Check sheet for the modelled part. Datum: model origin and axes. Units: mm. Face numbers are marked on the shaded views. A direction names the side the tool comes from. Round coordinates to 2 decimals unless told otherwise and drop trailing zeros. Order: outer loops, then holes, each group sorted by start corner. A loop starts at its lowest first (then second) coordinate and runs counter-clockwise, first axis right, second up.
(1) Mould release check, pull along X, two halves, no side actions. Record for the marked faces 3, 4 and 5: released by +X, released by -X, zero draft, split by the parting line, or undercut.
(2) Sectioned sample at A-A, the plane y = 6.25. Enter the section's corners in (x, z), and give its area (3 significant figures).
(3) Thickness scan on probe 1 along X at (y, z) = (2.5, -17); probe 2 along Y at (x, z) = (28.25, -22.5); probe 3 along X at (y, z) = (0.75, -21.75). Record the ranges inside material, lowest first.
(4) Sectioned sample at B-B, the plane z = -7.75. Enter the section's corners in (x, y).
(5) Depth check by flat-ended pin: pin 1 (4.5 mm diameter, centred on x = 23.5, z = -9, fed in from +Y); pin 2 (1 mm diameter, centred on y = 0.5, z = -18, fed in from +X); pin 3 (0.6 mm diameter, centred on x = 31, z = -19, fed in from -Y). Enter the tip coordinate at first touch or a pass-through.
(6) Tool access check on the marked faces 1 and 2. Record the directions out of +Z, -Z, +X, -X, +Y, -Y that give a thin tool (end or side, any length) a straight path to the whole face; none if there is none.
(7) Sectioned sample at C-C, the plane x = 25.75. Enter the section's corners in (y, z).
(8) Sectioned sample at D-D, the plane z = -22. Enter the section's corners in (x, y), and give its area (3 significant figures).
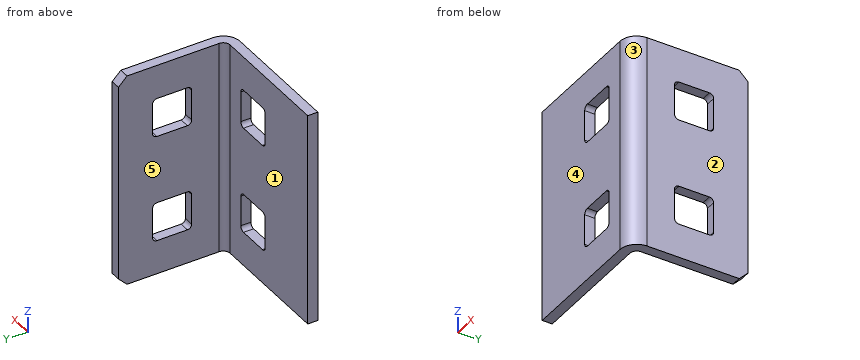
Autodesk Inventor part; units mm, degrees
ref_plane "Flange Pattern Plane" through (31.75, 7.5406, -4.5466) normal (0, 1, 0) x (1, 0, 0)
ref_plane "YZ Plane" through (0, 0, 0) normal (1, 0, 0) x (0, 1, 0)
ref_plane "XZ Plane" through (0, 0, 0) normal (0, 1, 0) x (-1, 0, 0)
sketch "Sketch1" plane through (0, 0, 0) normal (0, 1, 0) x (-1, 0, 0)
  line L0 (-31.75, 0) -> (31.75, 0)
  line L1 (31.75, 0) -> (31.75, -25.4)
  line L2 (31.75, -25.4) -> (-31.75, -25.4)
  line L3 (-31.75, -25.4) -> (-31.75, 0)
  line L4 (31.75, 0) -> (-31.75, -25.4) construction
  point P0 (0, 0)
  point P1 (0, 0)
  dimension "d0" = 63.5
  dimension "d1" = 25.4
extrude "Plate1" add sketch "Sketch1" along normal blind 1.1906
sketch "Sketch2" plane through (30.5594, 0, -25.4) normal (1, 0, 0) x (0, 1, 0)
  line L0 (0, 25.4) -> (0, 0)
  line L1 (0, 0) -> (13.8906, 0)
  line L2 (13.8906, 0) -> (13.8906, 25.4)
  line L3 (13.8906, 25.4) -> (0, 25.4)
edge flange "Flanges" height 12.7 angle 90 thickness 1.1906 bend radius 0.7937 thickness toward (1, 0, 0) relief tear relief width 1.1906 relief depth 0.5953 corner gap 1.1906 corner form 0 edges at (31.75, 1.1906, -12.7) (-31.75, 1.1906, -12.7) wall of the first edge with corners at (30.5594, 0, 0) (30.5594, 0, -25.4) (30.5594, 13.8906, -25.4) (30.5594, 13.8906, 0)
bend "Bend1"
corner "Corner1"
sketch "Sketch3" plane through (31.75, 1.9844, -25.4) normal (1, 0, 0) x (0, 0, -1)
  line L0 (-20.8534, 7.8676) -> (-17.2466, 7.8676)
  line L1 (-16.7386, 7.3596) -> (-16.7386, 3.7528)
  line L2 (-17.2466, 3.2448) -> (-20.8534, 3.2448)
  line L3 (-21.3614, 3.7528) -> (-21.3614, 7.3596)
  arc A0 (-20.8534, 7.8676) -> (-21.3614, 7.3596) centre (-20.8534, 7.3596) ccw
  arc A1 (-16.7386, 7.3596) -> (-17.2466, 7.8676) centre (-17.2466, 7.3596) ccw
  arc A2 (-17.2466, 3.2448) -> (-16.7386, 3.7528) centre (-17.2466, 3.7528) ccw
  arc A3 (-21.3614, 3.7528) -> (-20.8534, 3.2448) centre (-20.8534, 3.7528) ccw
  line L4 (-25.4, 0) -> (-25.4, 11.9062) construction
  line L5 (-25.4, 11.9062) -> (0, 11.9063) construction
  line L6 (-20.8534, 7.3596) -> (-17.2466, 3.7528) construction
  point P0 (-25.4, -1.9844)
  point P1 (-16.7386, 3.2448)
  point P2 (-21.3614, 3.2448)
  point P3 (-19.05, 5.5562)
  dimension "d16" = 4.6228
  dimension "d17" = 0.508
  dimension "d20" = 6.35
  dimension "d21" = 6.35
extrude "Flange Stamp" cut sketch "Sketch3" against normal blind 1.1906
sketch "Sketch7" plane through (31.75, 1.9844, 0) normal (1, 0, 0) x (0, 0, -1)
  arc A0 (4.5466, 7.8676) -> (4.0386, 7.3596) centre (4.5466, 7.3596) ccw construction
  arc A1 (8.1534, 3.2448) -> (8.6614, 3.7528) centre (8.1534, 3.7528) ccw construction
  circle A2 centre (6.35, 5.5563) radius 2.1844
  line L0 (4.5466, 7.3596) -> (8.1534, 3.7528) construction
  point P0 (0, -1.9844)
  dimension "d46" = 4.3688
surface extrude "Flange Circle" sketch "Sketch7" against normal up to surface (1.1906 mm away) shown yes curves A2
ref_plane "Flange Pattern Plane" through (31.75, 7.5406, -4.5466) normal (0, 1, 0) x (1, 0, 0)
sketch "Flange Pattern Sketch" plane through (31.75, 7.5406, -4.5466) normal (0, 1, 0) x (1, 0, 0)
  line L0 (0, 3.6068) -> (0, 0) construction
  line L1 (-76.2822, -4.5466) -> (13.1932, -4.5466) construction
  line L2 (0, 0) -> (-1.1906, 0) construction
  point P0 (-31.75, -4.5466)
  point P1 (0, 1.8034)
  point P2 (0, 14.5034)
  dimension "d131" = 12.7
  dimension "d134" = 12.7
pattern_sketch "Flange Pattern" of "Flange Circle", "Flange Stamp" from (31.75, 7.5406, -6.35) copies at (31.75, 7.5406, -19.05)
sketch "Sketch8" plane through (0, 0, 0) normal (0, -1, 0) x (1, 0, 0)
  line L0 (29.7656, 0) -> (-29.7656, 0) construction
  line L1 (27.2034, -4.0386) -> (23.5966, -4.0386)
  line L2 (23.0886, -4.5466) -> (23.0886, -8.1534)
  line L3 (23.5966, -8.6614) -> (27.2034, -8.6614)
  line L4 (27.7114, -8.1534) -> (27.7114, -4.5466)
  arc A0 (27.7114, -4.5466) -> (27.2034, -4.0386) centre (27.2034, -4.5466) ccw
  arc A1 (27.2034, -8.6614) -> (27.7114, -8.1534) centre (27.2034, -8.1534) ccw
  arc A2 (23.0886, -8.1534) -> (23.5966, -8.6614) centre (23.5966, -8.1534) ccw
  arc A3 (23.5966, -4.0386) -> (23.0886, -4.5466) centre (23.5966, -4.5466) ccw
  line L5 (27.2034, -4.5466) -> (23.5966, -8.1534) construction
  line L6 (31.75, 0) -> (31.75, -25.4) construction
  point P0 (0, 0)
  point P1 (23.0886, -8.6614)
  point P2 (27.7114, -8.6614)
  point P3 (25.4, -6.35)
  dimension "d49" = 4.6228
  dimension "d50" = 0.508
  dimension "d51" = 6.35
  dimension "d52" = 6.35
extrude "Body Stamp" cut sketch "Sketch8" against normal blind 1.1906
sketch "Sketch9" plane through (0, 0, 0) normal (0, -1, 0) x (1, 0, 0)
  arc A0 (27.7114, -4.5466) -> (27.2034, -4.0386) centre (27.2034, -4.5466) ccw construction
  arc A1 (23.0886, -8.1534) -> (23.5966, -8.6614) centre (23.5966, -8.1534) ccw construction
  line L0 (27.2034, -4.5466) -> (23.5966, -8.1534) construction
  circle A2 centre (25.4, -6.35) radius 2.1844
  point P0 (0, 0)
  dimension "d55" = 4.3688
surface extrude "Body Circle" sketch "Sketch9" against normal up to surface (1.1906 mm away) shown yes curves A2
sketch "Body Pattern Sketch" plane through (0, 0, 0) normal (0, -1, 0) x (1, 0, 0)
  line L0 (29.7656, 0) -> (-29.7656, 0) construction
  line L1 (31.75, 0) -> (31.75, -25.4) construction
  circle A0 centre (25.4, -6.35) radius 2.1844 construction
  point P0 (0, 0)
  point P1 (25.4, -19.05)
  dimension "d62" = 12.7
  dimension "d65" = 12.7
  dimension "d139" = 12.7
pattern_sketch "Body Pattern" of "Body Stamp", "Body Circle" from (25.4, 0, -6.35) copies at (25.4, 0, -19.05)
sketch "Arc Length" plane through (30.5594, 1.9844, 0) normal (0, 0, 1) x (1, 0, 0)
  line L0 (0, 0) -> (1.1906, 0) construction
  arc A0 (-0.7938, -0.7938) -> (0, 0) centre (-0.7938, 0) ccw construction
  line L1 (-0.7938, -1.9844) -> (-0.7938, -0.7938) construction
  arc A1 (-0.7938, -1.9844) -> (1.1906, 0) centre (-0.7938, 0) ccw construction
  point P0 (-30.5594, -1.9844)
  dimension "d85" = 3.117
  dimension "d92" = 1.2468
sketch "Sketch13" plane through (31.75, 13.8906, 0) normal (1, 0, 0) x (0, 0, -1)
  line L0 (0, 0) -> (25.4, 0) construction
  line L1 (62.4078, 0) -> (63.4238, -1.016)
  line L2 (63.4238, -1.016) -> (64.4398, 0)
  line L3 (62.4078, 0) -> (64.4398, 0)
  line L4 (25.4, -11.9063) -> (0, -11.9063) construction
  line L5 (63.4238, -10.8903) -> (61.3168, -12.9972)
  line L6 (61.3168, -12.9972) -> (63.4238, -15.1042)
  line L7 (63.4238, -15.1042) -> (65.5308, -12.9972)
  line L8 (65.5308, -12.9972) -> (63.4238, -10.8903)
  line L9 (63.4238, -10.8903) -> (63.4238, -15.1042) construction
  line L10 (63.4238, -1.016) -> (63.4238, -10.8903) construction
  line L11 (0, -11.9063) -> (25.4, -11.9063) construction
  point P0 (0, -13.8906)
  dimension "d86" = 4.2139
  dimension "d88" = 1.016
  dimension "d91" = 1.016
  dimension "d102" = 63.4238
feature "Notch" [suppressed]
mirror "Notch Mirror" [suppressed]
pattern_linear "Notch Pattern" [suppressed]
chamfer "End Chamfer" distance 1.016 angle 45 4 edges at (-31.1547, 13.8906, -25.4) (31.1547, 13.8906, -25.4) (-31.1547, 13.8906, 0) (31.1547, 13.8906, 0)
sketch "Sketch14" plane through (-31.75, 1.9844, 419.1) normal (1, 0, 0) x (0, 0, -1)
  line L0 (419.1, 11.9063) -> (444.5, 11.9063) construction
  line L1 (419.1, 0) -> (419.1, 11.9063) construction
  line L2 (419.1, -1.9844) -> (444.5, -1.9844) construction
  line L3 (419.1, 11.9063) -> (444.5, 11.9063)
  line L4 (444.5, 11.9063) -> (444.5, -1.9844)
  line L5 (444.5, -1.9844) -> (419.1, -1.9844)
  line L6 (419.1, -1.9844) -> (419.1, 11.9063)
  point P0 (382.0521, -1.9844)
extrude "Half Cut" cut sketch "Sketch14" along normal blind 46.7614
equation "\"d1\" = 1.27 * Length"
equation "\"d18\" = Thickness"
equation "\"d53\" = Thickness"
equation "\"d89\" = Thickness"
equation "\"d2\" = Thickness"
equation "\"d3\" = BendReliefWidth"
equation "\"d4\" = BendReliefDepth"
equation "\"d5\" = MinimumRemnant"
equation "\"d6\" = TransitionRadius"
equation "\"d10\" = CornerReliefSize"
equation "\"d11\" = GapSize"
equation "\"d12\" = JacobiRadiusSize"
equation "\"BendRadius\" = Thickness"
equation "\"BendReliefWidth\" = Thickness"
equation "\"BendReliefDepth\" = 0.5 * Thickness"
equation "\"CornerReliefSize\" = 4 * Thickness"
equation "\"MinimumRemnant\" = 2 * Thickness"
equation "\"TransitionRadius\" = BendRadius"
equation "\"JacobiRadiusSize\" = BendRadius"
equation "\"GapSize\" = Thickness"
properties part number "Alu C 1x3x1x35"
Derived:
1. face 3: released by +X
1. face 4: zero draft
1. face 5: released by -X
2. outline: (30.56, -25.4) - (31.75, -25.4) - (31.75, -21.36) - (30.56, -21.36) - close; (30.56, -16.74) - (31.75, -16.74) - (31.75, -8.66) - (30.56, -8.66) - close; (30.56, -4.04) - (31.75, -4.04) - (31.75, 0) - (30.56, 0) - close
2. area: 19.2 mm2
3. probe 1: x = 30.56 to 31.75
3. probe 2: y = 0 to 1.19
3. probe 3: x = 15.01 to 31.32
4. outline: (15.01, 0) - (23.09, 0) - (23.09, 1.19) - (15.01, 1.19) - close; (27.71, 0) - (29.77, 0) arc R1.98 ccw to (31.75, 1.98) - (31.75, 5.23) - (30.56, 5.23) - (30.56, 1.98) arc R0.79 cw to (29.77, 1.19) - (27.71, 1.19) - close; (30.56, 9.85) - (31.75, 9.85) - (31.75, 13.89) - (30.56, 13.89) - close
5. pin 1: stops at y = 1.19
5. pin 2: stops at x = 31.49
5. pin 3: stops at y = 0.23
6. face 1: +Z, -Z, -X, +Y
6. face 2: +Z, -Z, +X, +Y, -Y
7. outline: (0, -25.4) - (1.19, -25.4) - (1.19, -21.36) - (0, -21.36) - close; (0, -16.74) - (1.19, -16.74) - (1.19, -8.66) - (0, -8.66) - close; (0, -4.04) - (1.19, -4.04) - (1.19, 0) - (0, 0) - close
8. outline: (15.01, 0) - (29.77, 0) arc R1.98 ccw to (31.75, 1.98) - (31.75, 13.89) - (30.56, 13.89) - (30.56, 1.98) arc R0.79 cw to (29.77, 1.19) - (15.01, 1.19) - close
8. area: 34.3 mm2
